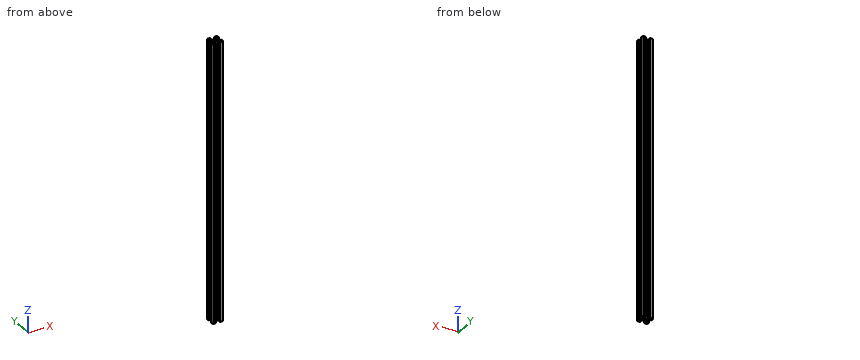
from build123d import *

# Parameters (mm, degrees)
SKETCH1_R      = 2.1
EXTRUDE1_DEPTH = 262.95


with BuildPart() as part:
    # Sketch1 → Extrude1 (new, symmetric)
    with BuildSketch(Plane.XY):
        with BuildLine():
            Line((-3.900660172, 0), (-3.900660172, -2.84))
            Line((-3.900660172, -2.84), (-6.56, -5.499339828))
            Line((-6.56, -5.499339828), (-8.2, -5.499339828))
            Line((-8.2, -5.499339828), (-8.2, -2.84))
            Line((-8.2, -2.84), (-10, -4.64))
            Line((-10, -4.64), (-10, -8.2))
            ThreePointArc((-10, -8.2), (-9.472792206, -9.472792206), (-8.2, -10))
            Line((-8.2, -10), (-4.64, -10))
            Line((-4.64, -10), (-2.84, -8.2))
            Line((-2.84, -8.2), (-5.499339828, -8.2))
            Line((-5.499339828, -8.2), (-5.499339828, -6.56))
            Line((-5.499339828, -6.56), (-2.84, -3.900660172))
            Line((-2.84, -3.900660172), (0, -3.900660172))
            Line((0, -3.900660172), (2.84, -3.900660172))
            Line((2.84, -3.900660172), (5.499339828, -6.56))
            Line((5.499339828, -6.56), (5.499339828, -8.2))
            Line((5.499339828, -8.2), (2.84, -8.2))
            Line((2.84, -8.2), (4.64, -10))
            Line((4.64, -10), (8.2, -10))
            ThreePointArc((8.2, -10), (9.472792206, -9.472792206), (10, -8.2))
            Line((10, -8.2), (10, -4.64))
            Line((10, -4.64), (8.2, -2.84))
            Line((8.2, -2.84), (8.2, -5.499339828))
            Line((8.2, -5.499339828), (6.56, -5.499339828))
            Line((6.56, -5.499339828), (3.900660172, -2.84))
            Line((3.900660172, -2.84), (3.900660172, 0))
            Line((3.900660172, 0), (3.900660172, 2.84))
            Line((3.900660172, 2.84), (6.56, 5.499339828))
            Line((6.56, 5.499339828), (8.2, 5.499339828))
            Line((8.2, 5.499339828), (8.2, 2.84))
            Line((8.2, 2.84), (10, 4.64))
            Line((10, 4.64), (10, 8.2))
            ThreePointArc((10, 8.2), (9.472792206, 9.472792206), (8.2, 10))
            Line((8.2, 10), (4.64, 10))
            Line((4.64, 10), (2.84, 8.2))
            Line((2.84, 8.2), (5.499339828, 8.2))
            Line((5.499339828, 8.2), (5.499339828, 6.56))
            Line((5.499339828, 6.56), (2.84, 3.900660172))
            Line((2.84, 3.900660172), (0, 3.900660172))
            Line((0, 3.900660172), (-2.84, 3.900660172))
            Line((-2.84, 3.900660172), (-5.499339828, 6.56))
            Line((-5.499339828, 6.56), (-5.499339828, 8.2))
            Line((-5.499339828, 8.2), (-2.84, 8.2))
            Line((-2.84, 8.2), (-4.64, 10))
            Line((-4.64, 10), (-8.2, 10))
            ThreePointArc((-8.2, 10), (-9.472792206, 9.472792206), (-10, 8.2))
            Line((-10, 8.2), (-10, 4.64))
            Line((-10, 4.64), (-8.2, 2.84))
            Line((-8.2, 2.84), (-8.2, 5.499339828))
            Line((-8.2, 5.499339828), (-6.56, 5.499339828))
            Line((-6.56, 5.499339828), (-3.900660172, 2.84))
            Line((-3.900660172, 2.84), (-3.900660172, 0))
        make_face()
        Circle(SKETCH1_R, mode=Mode.SUBTRACT)
        Polygon((-8.2, -8.2), (-8.2, -6.569339828), (-7.63, -6.569339828), (-6.569339828, -7.63), (-6.569339828, -8.2), align=None, mode=Mode.SUBTRACT)
        Polygon((-8.2, 6.569339828), (-8.2, 8.2), (-6.569339828, 8.2), (-6.569339828, 7.63), (-7.63, 6.569339828), align=None, mode=Mode.SUBTRACT)
        Polygon((6.569339828, 8.2), (8.2, 8.2), (8.2, 6.569339828), (7.63, 6.569339828), (6.569339828, 7.63), align=None, mode=Mode.SUBTRACT)
        Polygon((8.2, -6.569339828), (8.2, -8.2), (6.569339828, -8.2), (6.569339828, -7.63), (7.63, -6.569339828), align=None, mode=Mode.SUBTRACT)
    extrude(amount=EXTRUDE1_DEPTH, both=True)


solid = part.part
Part model, mm, in its own coordinate system. Give positions to 0.01 mm unless a question says otherwise; leave off trailing zeros. Put each result on its own line as item: value. Start each with the question number.
1) Saw through at A-A (z = -67). State how many separate pieces and enclosed holes the cut face has, then the cut area to 3 significant figures.
2) Probe probe 1 along X at (y, z) = (7.75, 78.5); probe 2 along Y at (x, z) = (-7, 93); probe 3 along Y at (x, z) = (0, 63.5). List the from-to ranges inside material, lowest first.
3) Flat gauge pins, fed straight in: pin 1 (1.7 mm diameter, centred on y = -0.5, z = -15, fed in from -X); pin 2 (3 mm diameter, centred on y = 0.5, z = 113, fed in from +X); pin 3 (1.7 mm diameter, centred on x = -0.5, z = -63.5, fed in from -Y); pin 4 (2 mm diameter, centred on x = -1, y = 7, fed in from -Z) (3 decimals). Where does each tip first touch, or does it go through?
Numbers:
1. separate pieces: 1
1. enclosed holes: 5
1. area: 160 mm^2
2. probe 1: -10 to -8.2, -6.57 to -5.5, 5.5 to 6.57, 8.2 to 10
2. probe 2: -10 to -8.2, -7.2 to -5.5, 5.5 to 7.2, 8.2 to 10
2. probe 3: -3.9 to -2.1, 2.1 to 3.9
3. pin 1: x = -3.9
3. pin 2: x = 3.9
3. pin 3: y = -3.9
3. pin 4: through
